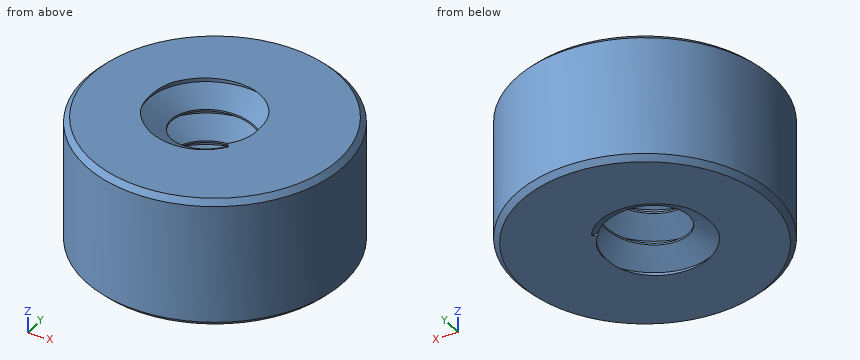
```python
from build123d import *

# Parameters (mm, degrees)
SKETCH1_R           = 6.35
SKETCH1_R_2         = 2.0447
BOSS_EXTRUDE1_DEPTH = 6.35
CUT_SWEEP1_PITCH    = 1.5875
CHAMFER1_SIZE       = 0.254


with BuildPart() as part:
    # Sketch1 → Boss-Extrude1 (new body)
    with BuildSketch(Plane.XY):
        Circle(SKETCH1_R)
        Circle(SKETCH1_R_2, mode=Mode.SUBTRACT)
    extrude(amount=BOSS_EXTRUDE1_DEPTH)

    # Cut-Sweep1: arcs per turn and ends read off the stored shape
    # Cut-Sweep1: the profile of Sketch2 profile screwed along a right-hand helix through 4.75 turns, 8 arcs to a turn; built about Z, then put on its axis
    cut_sweep1_z = Axis((0, 0, 0), (0, 0, 1))
    cut_sweep1_corners = [(2.0444, 0, -1.339811764), (3.175, 0, -0.68705955), (3.175, 0, -0.48862205), (2.0444, 0, 0.164130164)]
    with BuildLine(mode=Mode.PRIVATE) as cut_sweep1_profile:
        Line(cut_sweep1_corners[0], cut_sweep1_corners[1])
        Line(cut_sweep1_corners[1], cut_sweep1_corners[2])
        Line(cut_sweep1_corners[2], cut_sweep1_corners[3])
        Line(cut_sweep1_corners[3], cut_sweep1_corners[0])
    cut_sweep1_cap = Face(cut_sweep1_profile.wire())
    cut_sweep1_turn_angles = [0, 22.5, 45, 67.5, 90, 112.5, 135, 157.5, 180, 202.5, 225, 247.5, 270, 292.5, 315, 337.5, 360]
    cut_sweep1_turn_weights = [1, 0.9238795325112867, 1, 0.9238795325112867, 1, 0.9238795325112867, 1, 0.9238795325112867, 1, 0.9238795325112867, 1, 0.9238795325112867, 1, 0.9238795325112867, 1, 0.9238795325112867, 1]
    cut_sweep1_turn_rails = [Edge.make_bspline([Vector(p[0], p[1], 0).rotate(cut_sweep1_z, cut_sweep1_turn_angles[k]) / cut_sweep1_turn_weights[k] + Vector(0, 0, p[2] + CUT_SWEEP1_PITCH * cut_sweep1_turn_angles[k] / 360) for k in range(17)], [0, 0, 0, 1, 1, 2, 2, 3, 3, 4, 4, 5, 5, 6, 6, 7, 7, 8, 8, 8], 2, cut_sweep1_turn_weights) for p in cut_sweep1_corners]
    cut_sweep1_turn_sides = [Face.make_surface_from_curves(cut_sweep1_turn_rails[p[0]], cut_sweep1_turn_rails[p[1]]) for p in [(0, 1), (1, 2), (2, 3), (3, 0)]]
    cut_sweep1_last_angles = [1440, 1462.5, 1485, 1507.5, 1530, 1552.5, 1575, 1597.5, 1620, 1642.5, 1665, 1687.5, 1710]
    cut_sweep1_last_weights = [1, 0.9238795325112867, 1, 0.9238795325112867, 1, 0.9238795325112867, 1, 0.9238795325112867, 1, 0.9238795325112867, 1, 0.9238795325112769, 1]
    cut_sweep1_last_rails = [Edge.make_bspline([Vector(p[0], p[1], 0).rotate(cut_sweep1_z, cut_sweep1_last_angles[k]) / cut_sweep1_last_weights[k] + Vector(0, 0, p[2] + CUT_SWEEP1_PITCH * cut_sweep1_last_angles[k] / 360) for k in range(13)], [0, 0, 0, 1, 1, 2, 2, 3, 3, 4, 4, 5, 5, 6, 6, 6], 2, cut_sweep1_last_weights) for p in cut_sweep1_corners]
    cut_sweep1_last_sides = [Face.make_surface_from_curves(cut_sweep1_last_rails[p[0]], cut_sweep1_last_rails[p[1]]) for p in [(0, 1), (1, 2), (2, 3), (3, 0)]]
    cut_sweep1 = Plane(origin=(0, 0, 0), x_dir=(0.7071067811865512, 0.7071067811865438, 0), z_dir=(0, 0, 1)) * Solid(Shell([*[p.moved(Location((0, 0, CUT_SWEEP1_PITCH * i))) for i in range(4) for p in cut_sweep1_turn_sides], *cut_sweep1_last_sides, cut_sweep1_cap, cut_sweep1_cap.rotate(cut_sweep1_z, 1710).moved(Location((0, 0, CUT_SWEEP1_PITCH * 1710 / 360)))]))
    add(cut_sweep1, mode=Mode.SUBTRACT)

    # Chamfer1
    chamfer1_edges = [part.edges().sort_by_distance(p)[0] for p in [
        (-6.35, 0, 0),
        (-6.35, 0, 6.35),
    ]]
    chamfer(chamfer1_edges, length=CHAMFER1_SIZE)


solid = part.part
```
Work out the finished part from the listing and answer in its coordinate system (mm). Give positions to 0.01 mm unless a question says otherwise; leave off trailing zeros. Answer as CSV lines item,"result". Start each with the question number.
(1) Consider line 1 along Y through (x, z) = (0, 2) (3 decimals); line 2 along Y through (x, z) = (0.5, 4.5); line 3 along X through (y, z) = (1.75, 2.5). Determine where each line is inside the solid, lowest interval first.
(2) Section A-A, the plane y = 2.5 is taken. Give the number of separate pieces and of enclosed holes in the cut face, plus the area to 3 significant figures.
(3) Each of these flat-tipped pins is pushed along its axis until it touches: pin 1 Ø1 at (y, z) = (4, 3.5) entering from +X; pin 2 Ø1 at (x, z) = (-4, 2) entering from -Y; pin 3 Ø2.5 at (x, y) = (0, 0) entering from +Z. Where does it stop, or does it pass through?
Entries:
1,line 1,"-6.35 to -3.175, 2.045 to 6.35"
1,line 2,"-6.33 to -2.03, 3.02 to 6.33"
1,line 3,"-6.1 to -1.79, 2.65 to 6.1"
2,separate pieces,"1"
2,enclosed holes,"3"
2,area,"62.9 mm²"
3,pin 1,"x = 5.3"
3,pin 2,"y = -5.3"
3,pin 3,"through"
